```python
from build123d import *

# Parameters (mm, degrees)
SKETCH2_W                                         = 28
SKETCH2_H                                         = 28
BOSS_EXTRUDE1_DEPTH                               = 9.525
SKETCH6_W                                         = 12.7
SKETCH6_H                                         = 14.66469
CUT_EXTRUDE3_DEPTH                                = 9.525
FILLET1_R                                         = 2.38125
CSK_FOR_M2_5_FLAT_HEAD_MACHINE_SCREW1_D           = 2.9
CSK_FOR_M2_5_FLAT_HEAD_MACHINE_SCREW1_DEPTH       = 10.16
CSK_FOR_M2_5_FLAT_HEAD_MACHINE_SCREW1_CSINK_D     = 5.5
CSK_FOR_M2_5_FLAT_HEAD_MACHINE_SCREW1_CSINK_ANGLE = 90
CSK_FOR_M2_5_FLAT_HEAD_MACHINE_SCREW1_TIP         = 0.871247898


with BuildPart() as part:
    # Sketch2 → Boss-Extrude1 (new body)
    with BuildSketch(Plane(origin=(0, 0, 0), x_dir=(1, 0, 0), z_dir=(0, 1, 0))):
        Rectangle(SKETCH2_W, SKETCH2_H)
    extrude(amount=BOSS_EXTRUDE1_DEPTH)

    # Sketch6 → Cut-Extrude3 (cut)
    with BuildSketch(Plane(origin=(0, 9.525, 0), x_dir=(1, 0, 0), z_dir=(0, 1, 0))):
        Rectangle(SKETCH6_W, SKETCH6_H)
    extrude(amount=-CUT_EXTRUDE3_DEPTH, mode=Mode.SUBTRACT)

    # Fillet1
    fillet1_edges = [part.edges().sort_by_distance(p)[0] for p in [
        (-6.35, 4.7625, 7.332345),
        (-6.35, 4.7625, -7.332345),
        (6.35, 4.7625, -7.332345),
        (6.35, 4.7625, 7.332345),
    ]]
    fillet(fillet1_edges, radius=FILLET1_R)

    # CSK for M2.5 Flat Head Machine Screw1
    with Locations(Plane(origin=(0, 9.525, 0), x_dir=(1, 0, 0), z_dir=(0, 1, 0))):
        with Locations((-11, 0), (0, -11), (11, 0), (0, 11)):
            CounterSinkHole(CSK_FOR_M2_5_FLAT_HEAD_MACHINE_SCREW1_D / 2, CSK_FOR_M2_5_FLAT_HEAD_MACHINE_SCREW1_CSINK_D / 2, depth=CSK_FOR_M2_5_FLAT_HEAD_MACHINE_SCREW1_DEPTH, counter_sink_angle=CSK_FOR_M2_5_FLAT_HEAD_MACHINE_SCREW1_CSINK_ANGLE)
            with Locations((0, 0, -(CSK_FOR_M2_5_FLAT_HEAD_MACHINE_SCREW1_DEPTH + CSK_FOR_M2_5_FLAT_HEAD_MACHINE_SCREW1_TIP / 2))):  # 118° drill point
                Cone(0, CSK_FOR_M2_5_FLAT_HEAD_MACHINE_SCREW1_D / 2, CSK_FOR_M2_5_FLAT_HEAD_MACHINE_SCREW1_TIP, mode=Mode.SUBTRACT)


solid = part.part
```
The listing builds one solid part. Answer for the finished solid, in the listing's coordinates (mm). A direction names the side the tool comes from. Coordinates: 2 decimals unless noted, no trailing zeros. Write each loop counter-clockwise with the first axis right and the second up, starting at its lowest first coordinate (ties: lowest second). Pieces come first, ordered by that corner, then holes. Notation, with made-up numbers: (34, 64.25) -> (56, 64.25) arc R14 cw to (56, 68.25) -> close; hole circle Ø6 at (65, 23). An arc over 180 degrees is marked (long way). Write each question's results on one line, items separated by ' | '. Start each with the question number.
1) A cutting plane is placed at D-D (z = 11). Determine the outline of the cut face in (x, y) (3 decimals).
2) A cutting plane is placed at C-C (x = 0). Determine the outline of the cut face in (y, z) (3 decimals).
3) For a pull along Z with two mould halves and no side action, classify faces 1 (the flat face through (-6.4, 9.525, -6.4)), 2 (the flat face through (0, 5, 14)), 3 (the cylindrical face through (0.314, 4.055, 12.416)) as +Z half, -Z half, draft (parallel to the pull), parting line (faces both ways), or undercut.
4) Straight lines are drawn through the part: probe 1 along Z at (x, y) = (0, 3.5); probe 2 along X at (y, z) = (5.5, -11); probe 3 along Z at (x, y) = (-2.5, 8.5). For each, find the intervals that lie inside material, in ascending order.
5) A tool of negligible diameter and unlimited length cuts with its end or side. For faces 4 (the flat face through (6.35, 5, 0)), 5 (the flat face through (-6.4, 0, -6.4)), from which of +Z, -Z, +X, -X, +Y, -Y can it reach the whole face along a straight path? Write none if from no direction.
6) A cutting plane is placed at B-B (y = 1.75). Determine the outline of the cut face in (x, z), then the cut area to 3 significant figures.
7) A cutting plane is placed at A-A (z = 0). Determine the outline of the cut face in (x, y) (3 decimals).
Values follow:
1) outline: (-14, 0) -> (-1.45, 0) -> (-1.45, 8.225) -> (-2.75, 9.525) -> (-14, 9.525) -> close; (1.45, 0) -> (14, 0) -> (14, 9.525) -> (2.75, 9.525) -> (1.45, 8.225) -> close
2) outline: (0, -14) -> (9.525, -14) -> (9.525, -13.75) -> (8.225, -12.45) -> (0, -12.45) -> close; (0, -9.55) -> (8.225, -9.55) -> (9.525, -8.25) -> (9.525, -7.332) -> (0, -7.332) -> close; (0, 7.332) -> (9.525, 7.332) -> (9.525, 8.25) -> (8.225, 9.55) -> (0, 9.55) -> close; (0, 12.45) -> (8.225, 12.45) -> (9.525, 13.75) -> (9.525, 14) -> (0, 14) -> close
3) face 1: draft | face 2: +Z half | face 3: undercut
4) probe 1: -14 to -12.45, -9.55 to -7.33, 7.33 to 9.55, 12.45 to 14 | probe 2: -14 to -1.45, 1.45 to 14 | probe 3: -14 to -7.33, 7.33 to 14
5) face 4: +Y, -Y | face 5: +Z, -Z, +X, -X, -Y
6) outline: (-14, -14) -> (14, -14) -> (14, 14) -> (-14, 14) -> close; hole circle Ø2.9 at (-11, 0); hole (-6.35, -4.95) arc R2.38 ccw to (-3.97, -7.33) -> (3.97, -7.33) arc R2.38 ccw to (6.35, -4.95) -> (6.35, 4.95) arc R2.38 ccw to (3.97, 7.33) -> (-3.97, 7.33) arc R2.38 ccw to (-6.35, 4.95) -> close; hole circle Ø2.9 at (0, -11); hole circle Ø2.9 at (0, 11); hole circle Ø2.9 at (11, 0) | area: 576 mm²
7) outline: (-14, 0) -> (-12.45, 0) -> (-12.45, 8.225) -> (-13.75, 9.525) -> (-14, 9.525) -> close; (-9.55, 0) -> (-6.35, 0) -> (-6.35, 9.525) -> (-8.25, 9.525) -> (-9.55, 8.225) -> close; (6.35, 0) -> (9.55, 0) -> (9.55, 8.225) -> (8.25, 9.525) -> (6.35, 9.525) -> close; (12.45, 0) -> (14, 0) -> (14, 9.525) -> (13.75, 9.525) -> (12.45, 8.225) -> close
